Geometry check sheet. Reference: the model listing, model coordinates, mm. Round coordinates to 2 decimals unless told otherwise and drop trailing zeros. Loops run counter-clockwise (first coordinate to the right, second up) from the corner with the lowest first, then second, coordinate; pieces in that order, holes last. Notation, with made-up numbers: M -4,79 L 21,79 A5 cw 21,85 Z; hole C 3.25,67 d2. An arc over 180 degrees is marked long. Answer in a Markdown table with one row per item. Add a question column.
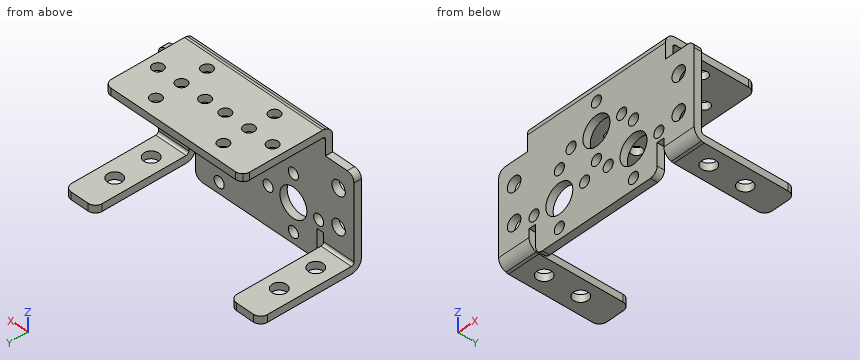
```python
from build123d import *

# Parameters (mm, degrees)
SKETCH1_R                    = 1.5
SKETCH1_R_2                  = 2
SKETCH1_R_3                  = 4
BASE_FLANGE1_DEPTH           = 2
SKETCHED_START               = -20.5
SKETCHED_BEND1_DEPTH         = 41
SKETCHED_START_2             = -29
SKETCHED_BEND1_2_DEPTH       = 9
SKETCHED_START_3             = 20
SKETCHED_BEND1_3_DEPTH       = 9
SKETCHED_BEND1_4_DEPTH       = 41
SKETCHED_BEND1_5_DEPTH       = 9
SKETCHED_BEND1_6_DEPTH       = 9
SKETCHED_START_4             = -26
SKETCHED_BEND1_7_OUTLINE_R   = 1.5
SKETCHED_BEND1_7_OUTLINE_R_2 = 2
SKETCHED_BEND1_7_DEPTH       = 33
SKETCHED_START_5             = 5
SKETCHED_BEND1_8_DEPTH       = 2


with BuildPart() as part:
    # Base-Flange1: sheet metal written as solids
    # Sketch1 → Base-Flange1 (new body)
    with BuildSketch(Plane(origin=(0, 0, 0), x_dir=(1, 0, 0), z_dir=(0, 1, 0))):
        with BuildLine():
            Line((-27, 0), (-20.5, 0))
            Line((-20.5, 0), (-20.5, -27))
            ThreePointArc((-20.5, -27), (-19.914213562, -28.414213562), (-18.5, -29))
            Line((-18.5, -29), (18.5, -29))
            ThreePointArc((18.5, -29), (19.914213562, -28.414213562), (20.5, -27))
            Line((20.5, -27), (20.5, 0))
            Line((20.5, 0), (27, 0))
            ThreePointArc((27, 0), (28.414213562, 0.585786438), (29, 2))
            Line((29, 2), (29, 48))
            ThreePointArc((29, 48), (28.414213562, 49.414213562), (27, 50))
            Line((27, 50), (22, 50))
            ThreePointArc((22, 50), (20.585786438, 49.414213562), (20, 48))
            Line((20, 48), (20, 20))
            Line((20, 20), (18, 20))
            Line((18, 20), (18, 26))
            ThreePointArc((18, 26), (17.414213562, 27.414213562), (16, 28))
            Line((16, 28), (-16, 28))
            ThreePointArc((-16, 28), (-17.414213562, 27.414213562), (-18, 26))
            Line((-18, 26), (-18, 20))
            Line((-18, 20), (-20, 20))
            Line((-20, 20), (-20, 48))
            ThreePointArc((-20, 48), (-20.585786438, 49.414213562), (-22, 50))
            Line((-22, 50), (-27, 50))
            ThreePointArc((-27, 50), (-28.414213562, 49.414213562), (-29, 48))
            Line((-29, 48), (-29, 2))
            ThreePointArc((-29, 2), (-28.414213562, 0.585786438), (-27, 0))
        make_face()
        with Locations(Location((-17, -17.5, 0), (0, 0, 270))):
            Circle(SKETCH1_R, mode=Mode.SUBTRACT)
        with Locations(Location((-10, -17.5, 0), (0, 0, 270))):
            Circle(SKETCH1_R, mode=Mode.SUBTRACT)
        with Locations(Location((-10, -10.5, 0), (0, 0, 270))):
            Circle(SKETCH1_R, mode=Mode.SUBTRACT)
        with Locations(Location((-3, -17.5, 0), (0, 0, 270))):
            Circle(SKETCH1_R, mode=Mode.SUBTRACT)
        with Locations(Location((-10, -24.5, 0), (0, 0, 270))):
            Circle(SKETCH1_R, mode=Mode.SUBTRACT)
        with Locations(Location((24.4, 40.5, 0), (0, 0, 270))):
            Circle(SKETCH1_R_2, mode=Mode.SUBTRACT)
        with Locations(Location((24.4, 30.5, 0), (0, 0, 270))):
            Circle(SKETCH1_R_2, mode=Mode.SUBTRACT)
        with Locations(Location((-24.4, 30.5, 0), (0, 0, 90))):
            Circle(SKETCH1_R_2, mode=Mode.SUBTRACT)
        with Locations(Location((-24.4, 40.5, 0), (0, 0, 90))):
            Circle(SKETCH1_R_2, mode=Mode.SUBTRACT)
        with Locations(Location((24.4, 6, 0), (0, 0, 270))):
            Circle(SKETCH1_R_2, mode=Mode.SUBTRACT)
        with Locations(Location((24.4, 16, 0), (0, 0, 270))):
            Circle(SKETCH1_R_2, mode=Mode.SUBTRACT)
        with Locations(Location((-24.4, 16, 0), (0, 0, 90))):
            Circle(SKETCH1_R_2, mode=Mode.SUBTRACT)
        with Locations(Location((-24.4, 6, 0), (0, 0, 90))):
            Circle(SKETCH1_R_2, mode=Mode.SUBTRACT)
        with Locations(Location((0, -1, 0), (0, 0, 270))):
            Circle(SKETCH1_R, mode=Mode.SUBTRACT)
        with Locations(Location((0, 6.5, 0), (0, 0, 270))):
            Circle(SKETCH1_R_3, mode=Mode.SUBTRACT)
        with Locations(Location((-7.5, 6.5, 0), (0, 0, 270))):
            Circle(SKETCH1_R, mode=Mode.SUBTRACT)
        with Locations(Location((0, 14, 0), (0, 0, 270))):
            Circle(SKETCH1_R, mode=Mode.SUBTRACT)
        with Locations(Location((7.5, 6.5, 0), (0, 0, 270))):
            Circle(SKETCH1_R, mode=Mode.SUBTRACT)
        with Locations(Location((-3.5, 17.5, 0), (0, 0, 270))):
            Circle(SKETCH1_R, mode=Mode.SUBTRACT)
        with Locations(Location((-11, 17.5, 0), (0, 0, 270))):
            Circle(SKETCH1_R_3, mode=Mode.SUBTRACT)
        with Locations(Location((-11, 25, 0), (0, 0, 270))):
            Circle(SKETCH1_R, mode=Mode.SUBTRACT)
        with Locations(Location((-18.5, 17.5, 0), (0, 0, 270))):
            Circle(SKETCH1_R, mode=Mode.SUBTRACT)
        with Locations(Location((-11, 10, 0), (0, 0, 270))):
            Circle(SKETCH1_R, mode=Mode.SUBTRACT)
        with Locations(Location((3.5, 17.5, 0), (0, 0, 270))):
            Circle(SKETCH1_R, mode=Mode.SUBTRACT)
        with Locations(Location((11, 17.5, 0), (0, 0, 270))):
            Circle(SKETCH1_R_3, mode=Mode.SUBTRACT)
        with Locations(Location((11, 10, 0), (0, 0, 270))):
            Circle(SKETCH1_R, mode=Mode.SUBTRACT)
        with Locations(Location((18.5, 17.5, 0), (0, 0, 270))):
            Circle(SKETCH1_R, mode=Mode.SUBTRACT)
        with Locations(Location((11, 25, 0), (0, 0, 270))):
            Circle(SKETCH1_R, mode=Mode.SUBTRACT)
        with Locations(Location((10, -10.5, 0), (0, 0, 90))):
            Circle(SKETCH1_R, mode=Mode.SUBTRACT)
        with Locations(Location((10, -24.5, 0), (0, 0, 90))):
            Circle(SKETCH1_R, mode=Mode.SUBTRACT)
        with Locations(Location((3, -17.5, 0), (0, 0, 90))):
            Circle(SKETCH1_R, mode=Mode.SUBTRACT)
        with Locations(Location((10, -17.5, 0), (0, 0, 90))):
            Circle(SKETCH1_R, mode=Mode.SUBTRACT)
        with Locations(Location((17, -17.5, 0), (0, 0, 90))):
            Circle(SKETCH1_R, mode=Mode.SUBTRACT)
    extrude(amount=-BASE_FLANGE1_DEPTH)

    # Sketched Bend1: read off the stored shape, not the designer's step
    # Sketched Bend1 outline → Sketched Bend1 (cut)
    with BuildSketch(Plane.YZ.offset(SKETCHED_START)):
        with BuildLine():
            Line((-2, 29), (-2, 4.2634))
            ThreePointArc((-2, 4.2634), (-1.443395312, 5.917667209), (0, 6.899002398))
            Line((0, 6.899002398), (0, 29))
            Line((0, 29), (-2, 29))
        make_face()
    extrude(amount=SKETCHED_BEND1_DEPTH, mode=Mode.SUBTRACT)

    # Sketched Bend1 2 outline → Sketched Bend1 2 (cut)
    with BuildSketch(Plane.YZ.offset(SKETCHED_START_2)):
        with BuildLine():
            ThreePointArc((0, -24.899002398), (-1.443395312, -23.917667209), (-2, -22.2634))
            Line((-2, -22.2634), (-2, -50))
            Line((-2, -50), (0, -50))
            Line((0, -50), (0, -24.899002398))
        make_face()
    extrude(amount=SKETCHED_BEND1_2_DEPTH, mode=Mode.SUBTRACT)

    # Sketched Bend1 3 outline → Sketched Bend1 3 (cut)
    with BuildSketch(Plane.YZ.offset(SKETCHED_START_3)):
        with BuildLine():
            ThreePointArc((0, -24.899002398), (-1.443395312, -23.917667209), (-2, -22.2634))
            Line((-2, -22.2634), (-2, -50))
            Line((-2, -50), (0, -50))
            Line((0, -50), (0, -24.899002398))
        make_face()
    extrude(amount=SKETCHED_BEND1_3_DEPTH, mode=Mode.SUBTRACT)

    # Sketched Bend1 4 outline → Sketched Bend1 4 (add)
    with BuildSketch(Plane.YZ.offset(SKETCHED_START)):
        with BuildLine():
            ThreePointArc((0.7366, 7), (0.364854094, 6.974633029), (0, 6.899002398))
            Line((0, 6.899002398), (0, 4.2634))
            ThreePointArc((0, 4.2634), (0.215745145, 4.784254855), (0.7366, 5))
            Line((0.7366, 5), (22.745355099, 5))
            Line((22.745355099, 5), (22.745355099, 7))
            Line((22.745355099, 7), (0.7366, 7))
        make_face()
    extrude(amount=SKETCHED_BEND1_4_DEPTH)

    # Sketched Bend1 5 outline → Sketched Bend1 5 (add)
    with BuildSketch(Plane.YZ.offset(SKETCHED_START_2)):
        with BuildLine():
            Line((0, -22.2634), (0, -24.899002398))
            ThreePointArc((0, -24.899002398), (0.364854094, -24.974633029), (0.7366, -25))
            Line((0.7366, -25), (25.745355099, -25))
            Line((25.745355099, -25), (25.745355099, -23))
            Line((25.745355099, -23), (0.7366, -23))
            ThreePointArc((0.7366, -23), (0.215745145, -22.784254855), (0, -22.2634))
        make_face()
    extrude(amount=SKETCHED_BEND1_5_DEPTH)

    # Sketched Bend1 6 outline → Sketched Bend1 6 (add)
    with BuildSketch(Plane.YZ.offset(SKETCHED_START_3)):
        with BuildLine():
            Line((0, -22.2634), (0, -24.899002398))
            ThreePointArc((0, -24.899002398), (0.364854094, -24.974633029), (0.7366, -25))
            Line((0.7366, -25), (25.745355099, -25))
            Line((25.745355099, -25), (25.745355099, -23))
            Line((25.745355099, -23), (0.7366, -23))
            ThreePointArc((0.7366, -23), (0.215745145, -22.784254855), (0, -22.2634))
        make_face()
    extrude(amount=SKETCHED_BEND1_6_DEPTH)

    # Sketched Bend1 7 outline → Sketched Bend1 7 (cut)
    with BuildSketch(Plane.XY.offset(SKETCHED_START_4)):
        with BuildLine():
            ThreePointArc((-29, 23.745355099), (-28.414213562, 25.159568661), (-27, 25.745355099))
            Line((-27, 25.745355099), (-29, 25.745355099))
            Line((-29, 25.745355099), (-29, 23.745355099))
        make_face()
        with BuildLine():
            ThreePointArc((-22, 25.745355099), (-20.585786438, 25.159568661), (-20, 23.745355099))
            Line((-20, 23.745355099), (-20, 25.745355099))
            Line((-20, 25.745355099), (-22, 25.745355099))
        make_face()
        with BuildLine():
            Line((29, 25.745355099), (27, 25.745355099))
            ThreePointArc((27, 25.745355099), (28.414213562, 25.159568661), (29, 23.745355099))
            Line((29, 23.745355099), (29, 25.745355099))
        make_face()
        with BuildLine():
            Line((20, 25.745355099), (20, 23.745355099))
            ThreePointArc((20, 23.745355099), (20.585786438, 25.159568661), (22, 25.745355099))
            Line((22, 25.745355099), (20, 25.745355099))
        make_face()
        with BuildLine():
            Line((20, 22.745355099), (18.5, 22.745355099))
            ThreePointArc((18.5, 22.745355099), (19.322875656, 22.568230754), (20, 22.068230754))
            Line((20, 22.068230754), (20, 22.745355099))
        make_face()
        with BuildLine():
            Line((-20, 22.745355099), (-20, 22.068230754))
            ThreePointArc((-20, 22.068230754), (-19.322875656, 22.568230754), (-18.5, 22.745355099))
            Line((-18.5, 22.745355099), (-20, 22.745355099))
        make_face()
        with Locations((17, 11.245355099)):
            Circle(SKETCHED_BEND1_7_OUTLINE_R)
        with Locations((-10, 18.245355099)):
            Circle(SKETCHED_BEND1_7_OUTLINE_R)
        with Locations((-3, 11.245355099)):
            Circle(SKETCHED_BEND1_7_OUTLINE_R)
        with Locations((-10, 4.245355099)):
            Circle(SKETCHED_BEND1_7_OUTLINE_R)
        with Locations((-17, 11.245355099)):
            Circle(SKETCHED_BEND1_7_OUTLINE_R)
        with Locations((10, 11.245355099)):
            Circle(SKETCHED_BEND1_7_OUTLINE_R)
        with Locations((3, 11.245355099)):
            Circle(SKETCHED_BEND1_7_OUTLINE_R)
        with Locations((10, 18.245355099)):
            Circle(SKETCHED_BEND1_7_OUTLINE_R)
        with Locations((-10, 11.245355099)):
            Circle(SKETCHED_BEND1_7_OUTLINE_R)
        with Locations((10, 4.245355099)):
            Circle(SKETCHED_BEND1_7_OUTLINE_R)
        with Locations((24.4, 16.245355099)):
            Circle(SKETCHED_BEND1_7_OUTLINE_R_2)
        with Locations((24.4, 6.245355099)):
            Circle(SKETCHED_BEND1_7_OUTLINE_R_2)
        with Locations((-24.4, 6.245355099)):
            Circle(SKETCHED_BEND1_7_OUTLINE_R_2)
        with Locations((-24.4, 16.245355099)):
            Circle(SKETCHED_BEND1_7_OUTLINE_R_2)
    extrude(amount=SKETCHED_BEND1_7_DEPTH, mode=Mode.SUBTRACT)

    # Sketched Bend1 8 outline → Sketched Bend1 8 (cut)
    with BuildSketch(Plane.XY.offset(SKETCHED_START_5)):
        with BuildLine():
            Line((-20.5, 22.745355099), (-20.5, 20.745355099))
            ThreePointArc((-20.5, 20.745355099), (-20.370828693, 21.45246188), (-20, 22.068230754))
            Line((-20, 22.068230754), (-20, 22.745355099))
            Line((-20, 22.745355099), (-20.5, 22.745355099))
        make_face()
        with BuildLine():
            Line((20, 22.745355099), (20, 22.068230754))
            ThreePointArc((20, 22.068230754), (20.370828693, 21.45246188), (20.5, 20.745355099))
            Line((20.5, 20.745355099), (20.5, 22.745355099))
            Line((20.5, 22.745355099), (20, 22.745355099))
        make_face()
    extrude(amount=SKETCHED_BEND1_8_DEPTH, mode=Mode.SUBTRACT)


solid = part.part
```
1) Go/stop test with flat-tipped pins: pin 1 (3.5 mm diameter, centred on x = -18.5, z = -17.5, fed in from +Y); pin 2 (8 mm diameter, centred on x = -20, y = 4.5, fed in from -Z); pin 3 (6 mm diameter, centred on x = 5.5, y = 5, fed in from -Z); pin 4 (2.5 mm diameter, centred on x = 10, y = 4.25, fed in from -Z). Record where each tip stops, or that it passes through.
2) Thickness scan on L1, parallel to Y at x = -2, z = 3; L2, parallel to Z at x = -22.5, y = 17.25; L3, parallel to X at y = 15.25, z = 5.5. Record the ranges inside material, lowest first. Write a range as [from, to].
3) Cross-section at C-C, the plane y = 5. Record the boundary of the cut face in (x, z).
4) Cross-section at B-B, the plane y = 15. Record the boundary of the cut face in (x, z).
5) Cross-section at A-A, the plane z = 1. Record the boundary of the cut face in (x, y), plus the area to 3 significant figures.
Worked answers:
| question | item | result |
|---|---|---|
| 1 | pin 1 | stops at y = 0 |
| 1 | pin 2 | stops at z = -25 |
| 1 | pin 3 | stops at z = 5 |
| 1 | pin 4 | passes through |
| 2 | L1 | y = [-2, 0] |
| 2 | L2 | z = [-25, -23] |
| 2 | L3 | x = [-20.5, 20.5] |
| 3 | outline | M -29,-25 L -25.96,-25 L -25.96,-23 L -29,-23 Z; M -22.84,-25 L -20,-25 L -20,-23 L -22.84,-23 Z; M -20.5,5 L -11.3,5 L -11.3,7 L -20.5,7 Z; M -8.7,5 L 8.7,5 L 8.7,7 L -8.7,7 Z; M 11.3,5 L 20.5,5 L 20.5,7 L 11.3,7 Z; M 20,-25 L 22.84,-25 L 22.84,-23 L 20,-23 Z; M 25.96,-25 L 29,-25 L 29,-23 L 25.96,-23 Z |
| 4 | outline | M -29,-25 L -25.96,-25 L -25.96,-23 L -29,-23 Z; M -22.84,-25 L -20,-25 L -20,-23 L -22.84,-23 Z; M -20.5,5 L 20.5,5 L 20.5,7 L -20.5,7 Z; M 20,-25 L 22.84,-25 L 22.84,-23 L 20,-23 Z; M 25.96,-25 L 29,-25 L 29,-23 L 25.96,-23 Z |
| 5 | outline | M -20.5,-2 L -1.5,-2 L -1.5,0 L -20.5,0 Z; M 1.5,-2 L 20.5,-2 L 20.5,0 L 1.5,0 Z |
| 5 | area | 76.0 mm2 |
